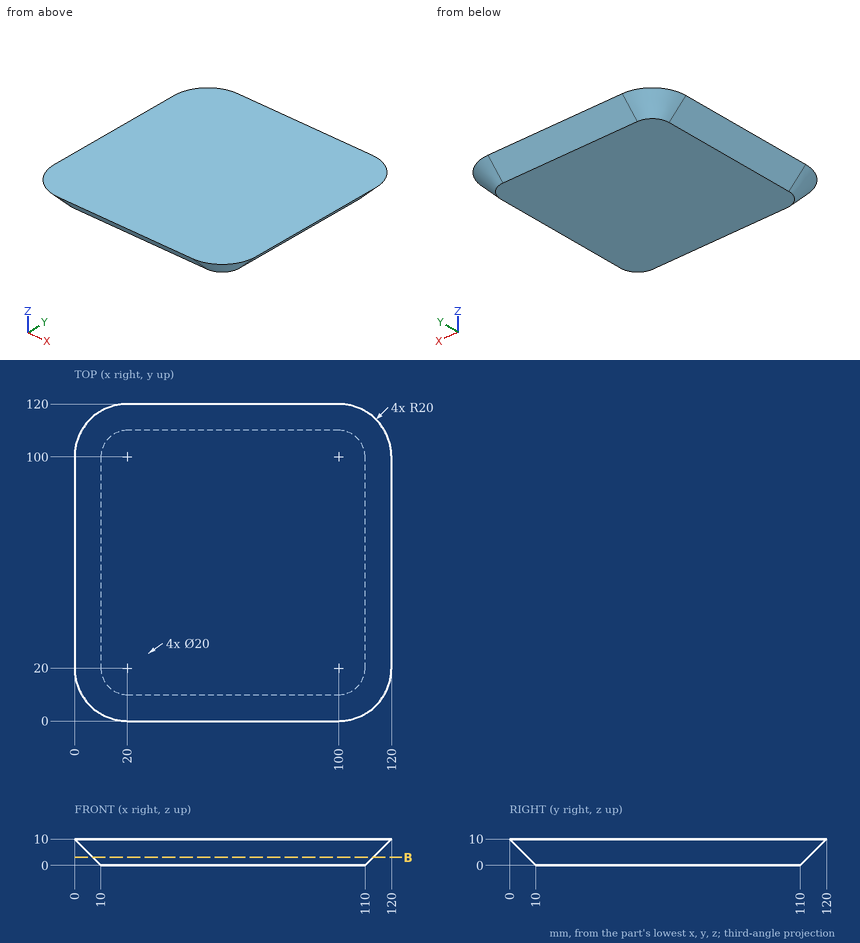
Job drawing, mm, ordinate dimensions from the low corner. One solid piece. Give positions to 0.01 mm unless a question says otherwise; leave off trailing zeros. Write each loop counter-clockwise with the first axis right and the second up, starting at its lowest first coordinate (ties: lowest second). Pieces come first, ordered by that corner, then holes. Notation, with made-up numbers: M 61.25,7.25 L 110.25,7.25 A20 cw 110.25,33.25 Z; hole C 81.5,-29 d3. An arc over 180 degrees is marked long. Put each result on its own line as item: value. Start each with the question number.
(1) Probe L1, parallel to Y at x = 46, z = 2.25; L2, parallel to Y at x = 8.5, z = 9.25; L3, parallel to X at y = 90, z = 6.5. List the from-to ranges inside material, lowest first.
(2) Flat gauge pins, fed straight in: pin 1 Ø1.5 at (y, z) = (95.5, 2) entering from -X; pin 2 Ø1 at (x, z) = (39.5, 5) entering from -Y; pin 3 Ø5 at (x, z) = (73, 7) entering from +Y. Where does each tip first touch, or does it go through?
(3) Band-saw the part on B-B, the plane z = 3. Write the cut outline in (x, y), and give its area (3 significant figures).
Response values:
1. L1: y = 7.75 to 112.25
1. L2: y = 4.56 to 115.44
1. L3: x = 3.5 to 116.5
2. pin 1: stops at x = 7.25
2. pin 2: stops at y = 4.5
2. pin 3: stops at y = 119.5
3. outline: M 7,20 A13 ccw 20,7 L 100,7 A13 ccw 113,20 L 113,100 A13 ccw 100,113 L 20,113 A13 ccw 7,100 Z
3. area: 11,100 mm2
